from build123d import *

# Parameters (mm, degrees)
SKETCH2_R           = 3.4925
BOSS_EXTRUDE1_DEPTH = 3.81
SKETCH3_R           = 2.413
CUT_EXTRUDE1_DEPTH  = 2.032
SKETCH4_R           = 1.143
CUT_EXTRUDE2_DEPTH  = 2.2225
SKETCH5_R           = 2.286
CUT_EXTRUDE3_DEPTH  = 1.016
SKETCH6_R           = 1.778
BOSS_EXTRUDE2_DEPTH = 1.4732


with BuildPart() as part:
    # Sketch2 → Boss-Extrude1 (new body)
    with BuildSketch(Plane.XY):
        with Locations(Location((0, 0, 0), (0, 0, 180))):
            Circle(SKETCH2_R)
    extrude(amount=BOSS_EXTRUDE1_DEPTH)

    # Sketch3 → Cut-Extrude1 (cut)
    with BuildSketch(Plane.XY.offset(3.81)):
        Circle(SKETCH3_R)
    extrude(amount=-CUT_EXTRUDE1_DEPTH, mode=Mode.SUBTRACT)

    # Sketch4 → Cut-Extrude2 (cut)
    with BuildSketch(Plane.XY.offset(1.778)):
        Circle(SKETCH4_R)
    extrude(amount=-CUT_EXTRUDE2_DEPTH, mode=Mode.SUBTRACT)

    # Sketch5 → Cut-Extrude3 (cut)
    with BuildSketch(Plane(origin=(0, 0, 0), x_dir=(-1, 0, 0), z_dir=(0, 0, -1))):
        Circle(SKETCH5_R)
    extrude(amount=-CUT_EXTRUDE3_DEPTH, mode=Mode.SUBTRACT)

    # Sketch6 → Boss-Extrude2 (add)
    with BuildSketch(Plane(origin=(0, 0, 0), x_dir=(-1, 0, 0), z_dir=(0, 0, -1))):
        with BuildLine():
            Line((0, 3.4925), (-13.006826988, 3.55595768))
            ThreePointArc((-13.006826988, 3.55595768), (-16.580175786, 0), (-13.006826988, -3.55595768))
            Line((-13.006826988, -3.55595768), (0, -3.4925))
            ThreePointArc((0, -3.4925), (-3.4925, 0), (0, 3.4925))
        make_face()
        with Locations((-13.97, 0)):
            Circle(SKETCH6_R, mode=Mode.SUBTRACT)
    extrude(amount=-BOSS_EXTRUDE2_DEPTH)


solid = part.part
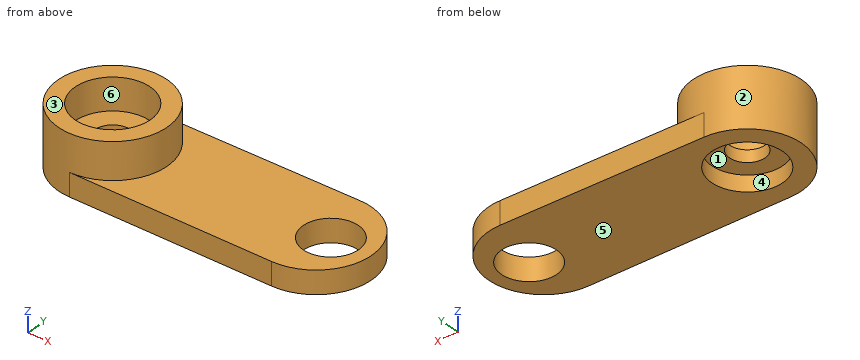
For this review, take the finished solid that the model builds, in its own axes (mm). Face numbers are marked on the shaded views. A direction names the side the tool comes from. Round coordinates to 2 decimals unless told otherwise and drop trailing zeros. Write each loop counter-clockwise with the first axis right and the second up, starting at its lowest first coordinate (ties: lowest second). Pieces come first, ordered by that corner, then holes. Notation, with made-up numbers: (63.25, -2) -> (112.25, -2) arc R33 ccw to (112.25, 35) -> close; hole circle Ø10 at (0, 51). An arc over 180 degrees is marked (long way). Use CSV: the item, a comma, the result in double quotes.
(1) For the marked faces 4, 5 and 6, list the 3-axis set-ups (+Z, -Z, +X, -X, +Y, -Y) from which the entire face can be reached by the end or side of a thin tool; tool diameter is ignored.
Computed values:
face 4,"-Z"
face 5,"-Z, +X, -X, +Y, -Y"
face 6,"+Z"
(2) Consider section C-C, the plane y = 0. Give the boundary of the cut face in (x, z), plus the area to 3 significant figures.
Computed values:
outline,"(-3.49, 0) -> (-2.29, 0) -> (-2.29, 1.02) -> (-1.14, 1.02) -> (-1.14, 1.78) -> (-2.41, 1.78) -> (-2.41, 3.81) -> (-3.49, 3.81) -> close; (1.14, 1.02) -> (2.29, 1.02) -> (2.29, 0) -> (12.19, 0) -> (12.19, 1.47) -> (3.49, 1.47) -> (3.49, 3.81) -> (2.41, 3.81) -> (2.41, 1.78) -> (1.14, 1.78) -> close; (15.75, 0) -> (16.58, 0) -> (16.58, 1.47) -> (15.75, 1.47) -> close"
area,"24.5 mm²"
(3) Consider section B-B, the plane x = 13.97. Give the boundary of the cut face in (y, z).
Computed values:
outline,"(-3.43, 0) -> (-1.78, 0) -> (-1.78, 1.47) -> (-3.43, 1.47) -> close; (1.78, 0) -> (3.43, 0) -> (3.43, 1.47) -> (1.78, 1.47) -> close"
(4) Consider section D-D, the plane z = 2. Give the boundary of the cut face in (x, y) (1 decimal).
Computed values:
outline,"circle Ø7 at (0, 0); hole circle Ø4.8 at (0, 0)"
(5) Clearance check with flat-ended pins moving along their axes: P1, Ø2.5, axis at x = 0, y = 0, coming from the -Z side; P2, Ø1.5, axis at x = 10, z = 3, coming from the +Y side; P3, Ø1, axis at x = 10, y = -0.5, coming from the -Z side; P4, Ø3, axis at x = 0, y = 0, coming from the +Z side. State where each tip first meets the part, or that it passes through.
Computed values:
P1,"z = 1.02"
P2,"through"
P3,"z = 0"
P4,"z = 1.78"
(6) Consider section A-A, the plane y = -1.5. Give the boundary of the cut face in (x, z), plus the area to 3 significant figures.
Computed values:
outline,"(-3.15, 0) -> (-1.73, 0) -> (-1.73, 1.02) -> (1.73, 1.02) -> (1.73, 0) -> (13.02, 0) -> (13.02, 1.47) -> (3.15, 1.47) -> (3.15, 3.81) -> (1.89, 3.81) -> (1.89, 1.78) -> (-1.89, 1.78) -> (-1.89, 3.81) -> (-3.15, 3.81) -> close; (14.92, 0) -> (16.25, 0) -> (16.25, 1.47) -> (14.92, 1.47) -> close"
area,"29.3 mm²"
(7) Draft analysis for pull direction Y (two halves, no side actions). For the marked faces 1, 2 and 3, state which applies: +Y half, -Y half, draft (parallel to the pull), parting line (faces both ways), or undercut.
Computed values:
face 1,"undercut"
face 2,"parting line"
face 3,"draft"
(8) To check wall thickness, follow L1, parallel to Y at x = 0, z = 2.5; L2, parallel to Z at x = 13.5, y = -2; L3, parallel to Y at x = 13.97, z = 0.8. State the ranges of each line that lie inside material, in increasing order. Write a range as [from, to].
Computed values:
L1,"[-3.49, -2.41], [2.41, 3.49]"
L2,"[0, 1.47]"
L3,"[-3.43, -1.78], [1.78, 3.43]"
